from build123d import *

# Parameters (mm, degrees)
F0_W     = 609.6
F0_H     = 609.6
F1_DEPTH = 304.8
F2_R     = 3.175
F3_DEPTH = 609.6
F5_DEPTH = 50.8
F7_DEPTH = 254
F8_W     = 127
F8_H     = 1.5291
F9_DEPTH = 25.4


with BuildPart() as f1:
    # F0 (on Top) → F1 (new body)
    with BuildSketch(Plane.XY):
        with Locations((8.20379, 40.765707)):
            Rectangle(F0_W, F0_H)
    extrude(amount=F1_DEPTH)

    # F2 (on face) → F3 (cut)
    with BuildSketch(Plane(origin=(-296.59621, 0, 0), x_dir=(0, -1, 0), z_dir=(-1, 0, 0))):
        with Locations((-329.690707, 15.875)):
            Circle(F2_R)
    extrude(amount=-F3_DEPTH, mode=Mode.SUBTRACT)

    # F4 (on face) → F5 (cut)
    with BuildSketch(Plane(origin=(-296.59621, 0, 0), x_dir=(0, -1, 0), z_dir=(-1, 0, 0))):
        with BuildLine():
            Line((143.384293, 19.05), (-301.115707, 19.05))
            ThreePointArc((-301.115707, 19.05), (-304.290707, 15.875), (-301.115707, 12.7))
            Line((-301.115707, 12.7), (143.384293, 12.7))
            ThreePointArc((143.384293, 12.7), (146.559293, 15.875), (143.384293, 19.05))
        make_face()
    extrude(amount=-F5_DEPTH, mode=Mode.SUBTRACT)

    # F6 (on face) → F7 (cut)
    with BuildSketch(Plane.XZ.offset(264.034293)):
        Polygon((254.007536, 300.3042), (209.278136, 304.8), (202.877336, 304.8), (158.147936, 300.3042), (158.147936, 292.7858), (254.007536, 292.7858), align=None)
        Polygon((-254.007536, 292.7858), (-158.147936, 292.7858), (-158.147936, 300.3042), (-202.877336, 304.8), (-209.278136, 304.8), (-254.007536, 300.3042), align=None)
        Polygon((24.286199, 295.275), (24.286199, 304.8), (-58.270179, 304.8), (-58.270179, 295.275), (-93.115404, 295.275), (-93.115404, 285.75), (62.347908, 285.75), (62.347908, 295.275), align=None)
    extrude(amount=-F7_DEPTH, mode=Mode.SUBTRACT)

    # F8 (on face) → F9 (cut)
    with BuildSketch(Plane.XY.offset(304.8)):
        with Locations((-194.99621, -260.882653)):
            Rectangle(F8_W, F8_H)
        with Locations((194.99621, -260.882653)):
            Rectangle(F8_W, F8_H)
    extrude(amount=-F9_DEPTH, mode=Mode.SUBTRACT)


solid = f1.part
CAD build for the part. Positions are in the model's coordinates, mm. A direction names the side the tool comes from. Give positions to 0.01 mm unless a question says otherwise; leave off trailing zeros. Write each loop counter-clockwise with the first axis right and the second up, starting at its lowest first coordinate (ties: lowest second). Pieces come first, ordered by that corner, then holes. Notation, with made-up numbers: (24.5, 78) - (75.5, 78) arc R12 cw to (75.5, 91) - close; hole circle Ø1 at (19, 36.5). An arc over 180 degrees is marked (long way). Put each result on its own line as item: value.
(1) Wall check: L1, parallel to Z at x = -247, y = -75.5; L2, parallel to Z at x = -270, y = 144.5; L3, parallel to Z at x = 4, y = -44.5. Give the ranges that are in metal, low to high.
Working result:
L1: 0 to 12.7, 19.05 to 292.79, 301.01 to 304.8
L2: 0 to 12.7, 19.05 to 304.8
L3: 0 to 285.75
(2) Saw through at C-C (y = -50). List the corners of the cut face in (x, z) (3 decimals), then the cut area to 3 significant figures.
Working result:
outline: (-296.596, 0) - (313.004, 0) - (313.004, 304.8) - (209.278, 304.8) - (254.008, 300.304) - (254.008, 292.786) - (158.148, 292.786) - (158.148, 300.304) - (202.877, 304.8) - (24.286, 304.8) - (24.286, 295.275) - (62.348, 295.275) - (62.348, 285.75) - (-93.115, 285.75) - (-93.115, 295.275) - (-58.27, 295.275) - (-58.27, 304.8) - (-202.877, 304.8) - (-158.148, 300.304) - (-158.148, 292.786) - (-254.008, 292.786) - (-254.008, 300.304) - (-209.278, 304.8) - (-296.596, 304.8) - (-296.596, 19.05) - (-245.796, 19.05) - (-245.796, 12.7) - (-296.596, 12.7) - close
area: 181,000 mm^2
(3) Saw through at B-B (x = -42). List the corners of the cut face in (y, z) (3 decimals), then the cut area to 3 significant figures.
Working result:
outline: (-264.034, 0) - (345.566, 0) - (345.566, 304.8) - (-10.034, 304.8) - (-10.034, 285.75) - (-264.034, 285.75) - close; hole circle Ø6.35 at (329.691, 15.875)
area: 181,000 mm^2
(4) Tool access for faces 1 (the flat face through (-196, -261.647, 289)), 2 (the flat face through (44, -139, 295.275)), 3 (the flat face through (-272, 76, 19.05)): list every direction of +Z, -Z, +X, -X, +Y, -Y with a clear straight run to the whole face (end or side of a thin tool).
Working result:
face 1: +Z
face 2: -Y
face 3: -X
(5) Saw through at A-A (y = -208). List the corners of the cut face in (x, z) (3 decimals).
Working result:
outline: (-296.596, 0) - (313.004, 0) - (313.004, 304.8) - (209.278, 304.8) - (254.008, 300.304) - (254.008, 292.786) - (158.148, 292.786) - (158.148, 300.304) - (202.877, 304.8) - (24.286, 304.8) - (24.286, 295.275) - (62.348, 295.275) - (62.348, 285.75) - (-93.115, 285.75) - (-93.115, 295.275) - (-58.27, 295.275) - (-58.27, 304.8) - (-202.877, 304.8) - (-158.148, 300.304) - (-158.148, 292.786) - (-254.008, 292.786) - (-254.008, 300.304) - (-209.278, 304.8) - (-296.596, 304.8) - close
(6) Pull direction Y, two halves, no side cores. Call faces 4 (the flat face through (-231.33, -136.827, 302.584)), 5 (the flat face through (4, -264.034, 150)), 6 (the flat face through (-196, -260.118, 289)): released by +Y, released by -Y, zero draft, split by the parting line, or undercut.
Working result:
face 4: zero draft
face 5: released by -Y
face 6: undercut
(7) Drop flat-ended pins along their axis: pin 1 Ø12 at (x, y) = (138, 44.5) entering from -Z; pin 2 Ø5.5 at (x, z) = (-18, 295.5) entering from -Y; pin 3 Ø1.5 at (x, y) = (10, -121) entering from +Z. Give the stop position or say it passes through.
Working result:
pin 1: z = 0
pin 2: y = -10.03
pin 3: z = 285.75
